Design review of the part built by this model. Coordinates are the model's own, in mm. Coordinates: 2 decimals unless noted, no trailing zeros. Write each loop counter-clockwise with the first axis right and the second up, starting at its lowest first coordinate (ties: lowest second). Pieces come first, ordered by that corner, then holes. Notation, with made-up numbers: (-27, 41) - (19, 41) arc R24 cw to (19, 80) - close; hole circle Ø1 at (-22, -11). An arc over 180 degrees is marked (long way). Use a Markdown table: item, result.
from build123d import *

# Parameters (mm, degrees)
SCHIZZO1_W                   = 24.5
SCHIZZO1_H                   = 22.0038
SCHIZZO1_R                   = 1
ESTRUSIONE_ESTRUSIONE1_DEPTH = 2
RACCORDO1_R                  = 3


with BuildPart() as part:
    # Schizzo1 → Estrusione-Estrusione1 (new body)
    with BuildSketch(Plane.XY):
        with Locations((10, 8.5)):
            Rectangle(SCHIZZO1_W, SCHIZZO1_H)
        Circle(SCHIZZO1_R, mode=Mode.SUBTRACT)
        with Locations((20, 0)):
            Circle(SCHIZZO1_R, mode=Mode.SUBTRACT)
        with Locations((20, 17)):
            Circle(SCHIZZO1_R, mode=Mode.SUBTRACT)
        with Locations((0, 17)):
            Circle(SCHIZZO1_R, mode=Mode.SUBTRACT)
    extrude(amount=ESTRUSIONE_ESTRUSIONE1_DEPTH)

    # Raccordo1
    raccordo1_edges = [part.edges().sort_by_distance(p)[0] for p in [
        (22.25, -2.5019, 1),
        (-2.25, -2.5019, 1),
        (-2.25, 19.5019, 1),
        (22.25, 19.5019, 1),
    ]]
    fillet(raccordo1_edges, radius=RACCORDO1_R)


solid = part.part
(1) For L1, parallel to Y at x = 0, z = 1.25; L2, parallel to X at y = 16.25, z = 1.5, list the stretches that pass through material, from the lowest coordinate up. Write a range as from..to.
Determined:
| item | result |
|---|---|
| L1 | -2.41..-1, 1..16, 18..19.41 |
| L2 | -2.25..-0.66, 0.66..19.34, 20.66..22.25 |
(2) Take a section at B-B on x = 20. Write out the cut boundary in (y, z).
Determined:
| item | result |
|---|---|
| outline | (-2.41, 0) - (-1, 0) - (-1, 2) - (-2.41, 2) - close; (1, 0) - (16, 0) - (16, 2) - (1, 2) - close; (18, 0) - (19.41, 0) - (19.41, 2) - (18, 2) - close |
(3) Take a section at C-C on y = 0. Write out the cut boundary in (x, z), and give its area (3 significant figures).
Determined:
| item | result |
|---|---|
| outline | (-2.21, 0) - (-1, 0) - (-1, 2) - (-2.21, 2) - close; (1, 0) - (19, 0) - (19, 2) - (1, 2) - close; (21, 0) - (22.21, 0) - (22.21, 2) - (21, 2) - close |
| area | 40.8 mm2 |
(4) Draft analysis for pull direction Y (two halves, no side actions). For faces 1 (the cylindrical face through (-1.395, 18.6, 1.014)), 2 (the flat face through (22.25, 8, 1)), 3 (the cylindrical face through (20, 16, 1)), state which applies: +Y half, -Y half, draft (parallel to the pull), parting line (faces both ways), or undercut.
Determined:
| item | result |
|---|---|
| face 1 | +Y half |
| face 2 | draft |
| face 3 | undercut |
(5) For pin 1 (1.2 mm diameter, centred on x = 0, y = 17, fed in from +Z), flat-tipped, find the tip position at first contact; note if it passes through.
Determined:
| item | result |
|---|---|
| pin 1 | through |
(6) Take a section at A-A on z = 1.6. Write out the cut boundary in (x, y), and give its area (3 significant figures).
Determined:
| item | result |
|---|---|
| outline | (-2.25, 0.5) arc R3 ccw to (0.75, -2.5) - (19.25, -2.5) arc R3 ccw to (22.25, 0.5) - (22.25, 16.5) arc R3 ccw to (19.25, 19.5) - (0.75, 19.5) arc R3 ccw to (-2.25, 16.5) - close; hole circle Ø2 at (0, 0); hole circle Ø2 at (0, 17); hole circle Ø2 at (20, 0); hole circle Ø2 at (20, 17) |
| area | 519 mm2 |
